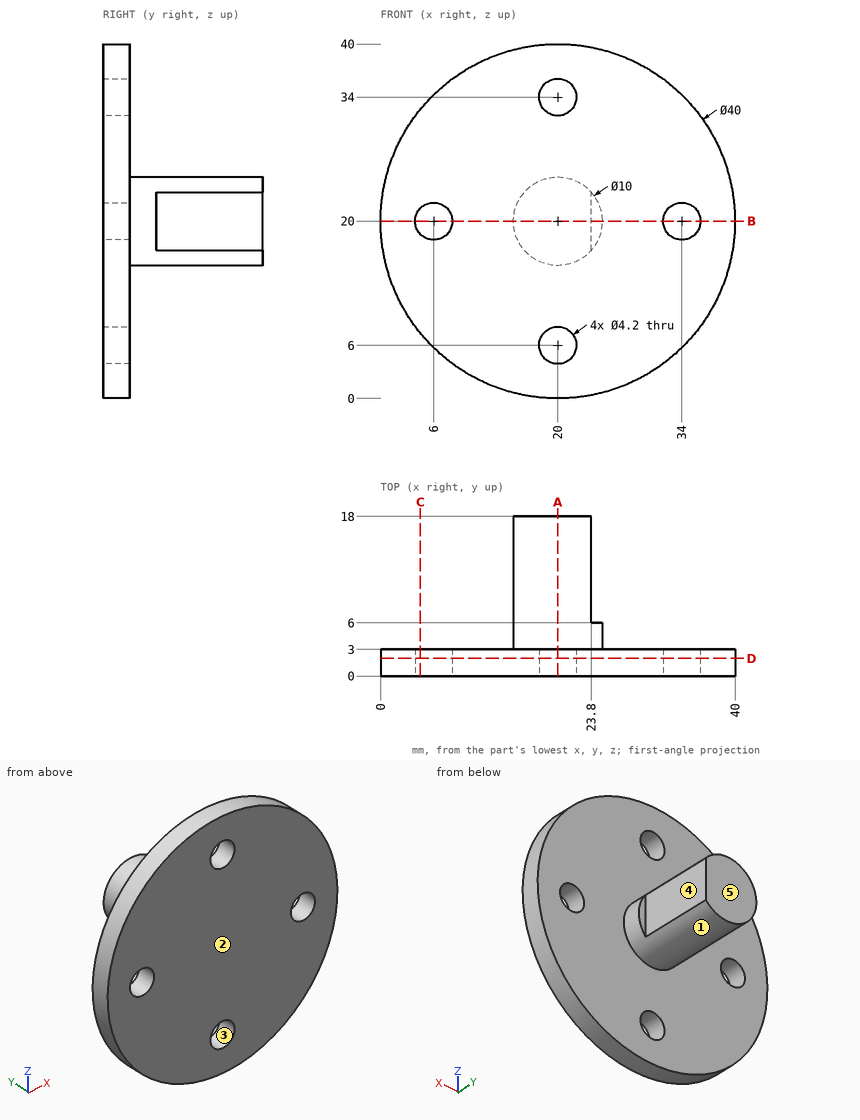
Geometry: see drawing. Coordinates: mm, zero at the bounding-box minimum. A direction names the side the tool comes from. Coordinates: 2 decimals unless noted, no trailing zeros. Loops run counter-clockwise (first coordinate to the right, second up) from the corner with the lowest first, then second, coordinate; pieces in that order, holes last. Notation, with made-up numbers: M 67,47 L 76,47 A21 cw 76,69 Z; hole C -31.75,84 d1. An arc over 180 degrees is marked long. Answer in a Markdown table with one row per item.
Q1. Section D-D on y = 2. Return the cut outline in (x, z), plus the area to 3 significant figures.
Answers below:
| item | result |
|---|---|
| outline | C 20,20 d40; hole C 6,20 d4.2; hole C 20,6 d4.2; hole C 20,34 d4.2; hole C 34,20 d4.2 |
| area | 1,200 mm^2 |
Q2. Section A-A on x = 20. Return the cut outline in (y, z).
Answers below:
| item | result |
|---|---|
| outline | M 0,0 L 3,0 L 3,3.9 L 0,3.9 Z; M 0,8.1 L 3,8.1 L 3,15 L 18,15 L 18,25 L 3,25 L 3,31.9 L 0,31.9 Z; M 0,36.1 L 3,36.1 L 3,40 L 0,40 Z |
Q3. Section B-B on z = 20. Return the cut outline in (x, y).
Answers below:
| item | result |
|---|---|
| outline | M 0,0 L 3.9,0 L 3.9,3 L 0,3 Z; M 8.1,0 L 31.9,0 L 31.9,3 L 25,3 L 25,6 L 23.8,6 L 23.8,18 L 15,18 L 15,3 L 8.1,3 Z; M 36.1,0 L 40,0 L 40,3 L 36.1,3 Z |
Q4. Ray query, probe 1 along X at (y, z) = (0.65, 20); probe 2 along Y at (x, z) = (23, 15); probe 3 along X at (y, z) = (1.9, 34). Return the intervals inside material, ascending. Write a range as from..to.
Answers below:
| item | result |
|---|---|
| probe 1 | x = 0..3.9, 8.1..31.9, 36.1..40 |
| probe 2 | y = 0..3 |
| probe 3 | x = 5.72..17.9, 22.1..34.28 |
Q5. Set-up query: the marked faces 1 and 2. Return all of +Z, -Z, +X, -X, +Y, -Y with unobstructed straight access to the full face (end or side cutting, diameter ignored); none if empty.
Answers below:
| item | result |
|---|---|
| face 1 | +Y |
| face 2 | +Z, -Z, +X, -X, -Y |
Q6. First-contact query: pin 1 (2.5 mm diameter, centred on x = 34, z = 20, fed in from +Y); pin 2 (8 mm diameter, centred on y = 4, z = 28.5, fed in from +X); pin 3 (8 mm diameter, centred on x = 31.5, z = 12, fed in from +Y); pin 4 (10 mm diameter, centred on y = 5, z = 11.5, fed in from +X). Flat tips, straight axial feed; report the tip coordinate or a pass-through.
Answers below:
| item | result |
|---|---|
| pin 1 | passes through |
| pin 2 | stops at x = 39.46 |
| pin 3 | stops at y = 3 |
| pin 4 | stops at x = 39.61 |
Q7. Draft query along X for the marked faces 3, 4 and 5. Return one class per face: pulls with the +X half, pulls with the -X half, needs draft (parallel to the pull), parting line crosses it, or undercut.
Answers below:
| item | result |
|---|---|
| face 3 | undercut |
| face 4 | pulls with the +X half |
| face 5 | needs draft |
Q8. Section C-C on x = 4.5. Return the cut outline in (y, z), plus the area to 3 significant figures.
Answers below:
| item | result |
|---|---|
| outline | M 0,7.36 L 3,7.36 L 3,18.53 L 0,18.53 Z; M 0,21.47 L 3,21.47 L 3,32.64 L 0,32.64 Z |
| area | 67.0 mm^2 |
